Geometry: see drawing. Coordinates: mm, zero at the bounding-box minimum. Coordinates: 2 decimals unless noted, no trailing zeros. Loops run counter-clockwise (first coordinate to the right, second up) from the corner with the lowest first, then second, coordinate; pieces in that order, holes last. Notation, with made-up numbers: (57.25, 7) - (62.25, 7) arc R26 cw to (62.25, 41) - close; hole circle Ø11 at (-17, 88). An arc over 180 degrees is marked (long way). Use one line per item in the form item = value.
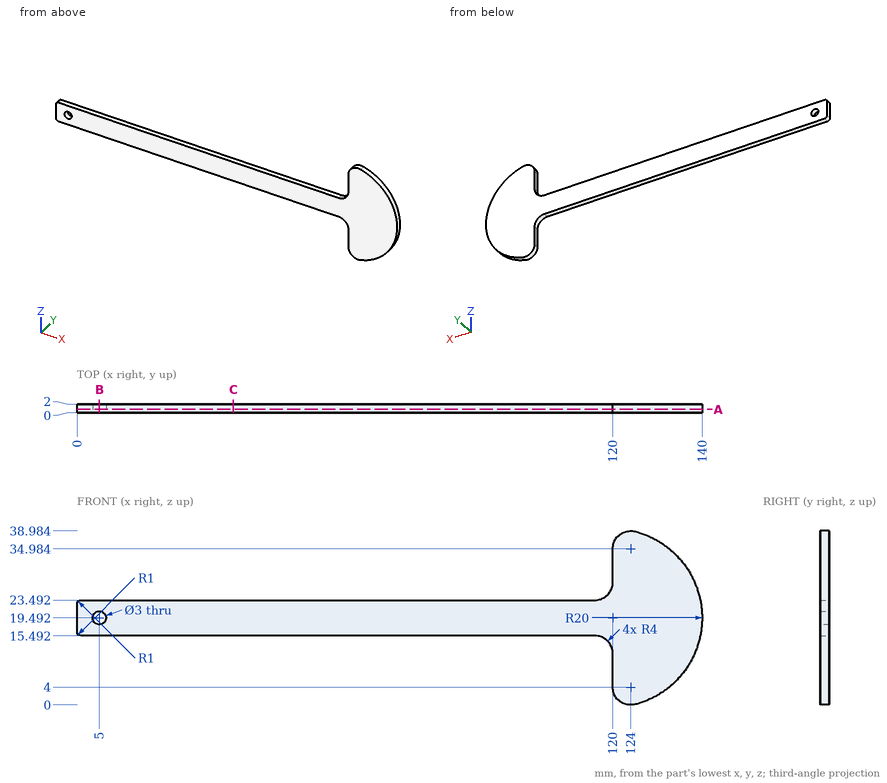
Q1. Cut plane B-B, the plane x = 5. Return loops of the section in (y, z), then the cut area to 3 significant figures.
Check values:
outline = (0, 15.49) - (2, 15.49) - (2, 17.99) - (0, 17.99) - close; (0, 20.99) - (2, 20.99) - (2, 23.49) - (0, 23.49) - close
area = 10.0 mm²
Q2. Cut plane C-C, the plane x = 35. Return loops of the section in (y, z).
Check values:
outline = (0, 15.49) - (2, 15.49) - (2, 23.49) - (0, 23.49) - close
Q3. Ray query, line 1 along Z through (x, y) = (5, 0.5); line 2 along Z through (x, y) = (69.5, 0.8); line 3 along X through (y, z) = (0.45, 13) (1 decimal). Return the intervals inside material, ascending. Write a range as [from, to].
Check values:
line_1 = [15.49, 17.99], [20.99, 23.49]
line_2 = [15.49, 23.49]
line_3 = [119.7, 138.9]
Q4. First-contact query: P1, Ø0.6, axis at y = 0.5, z = 32, coming from the -X side. Flat tip, straight axial feed; report the tip coordinate or a pass-through.
Check values:
P1 = 120
Q5. Cut plane A-A, the plane y = 0.8. Return loops of the section in (x, z), then the cut area to 3 significant figures.
Check values:
outline = (0, 16.49) arc R1 ccw to (1, 15.49) - (116, 15.49) arc R4 cw to (120, 11.49) - (120, 4) arc R4 ccw to (125, 0.13) arc R20 ccw to (125, 38.86) arc R4 ccw to (120, 34.98) - (120, 27.49) arc R4 cw to (116, 23.49) - (1, 23.49) arc R1 ccw to (0, 22.49) - close; hole circle Ø3 at (5, 19.49)
area = 1,580 mm²
